Autodesk Inventor part; units mm, degrees
ref_plane "YZ Plane" through (0, 0, 0) normal (1, 0, 0) x (0, 1, 0)
ref_plane "XZ Plane" through (0, 0, 0) normal (0, 1, 0) x (-1, 0, 0)
ref_plane "XY Plane" through (0, 0, 0) normal (0, 0, 1) x (1, 0, 0)
sketch "Sketch1" plane through (0, 0, 0) normal (1, 0, 0) x (0, 1, 0)
  line L0 (-30, 12.5) -> (30, 12.5)
  line L1 (30, 12.5) -> (30, -12.5)
  line L2 (30, -12.5) -> (-30, -12.5)
  line L3 (-30, -12.5) -> (-30, 12.5)
  line L4 (-30, 12.5) -> (30, -12.5) construction
  line L5 (30, 12.5) -> (-30, -12.5) construction
  line L6 (28, -10.5) -> (28, 10.5)
  line L7 (28, 10.5) -> (-28, 10.5)
  line L8 (-28, 10.5) -> (-28, -10.5)
  line L9 (-28, -10.5) -> (28, -10.5)
  point P0 (0, 0)
  dimension "d0" = 60
  dimension "d1" = 25
  dimension "d2" = 2
extrude "Extrusion1" add sketch "Sketch1" along normal blind 70
sketch "Sketch2" plane through (0, 30, 12.5) normal (0, 1, 0) x (1, 0, 0)
  circle A0 centre (15, 12.5) radius 2.75
  circle A1 centre (35, 12.5) radius 2.75
  circle A2 centre (55, 12.5) radius 2.75
  line L0 (0, 0) -> (0, 25)
  line L1 (15, 12.5) -> (55, 12.5) construction
  point P0 (0, 12.5)
  point P1 (0, 12.5)
  dimension "d5" = 5.5
  dimension "d6" = 5.5
  dimension "d7" = 5.5
  dimension "d8" = 20
  dimension "d9" = 20
  dimension "d10" = 15
  dimension "d11" = 40
extrude "Extrusion2" cut sketch "Sketch2" against normal through all
sketch "Sketch3" plane through (0, -30, 12.5) normal (0, 0, 1) x (1, 0, 0)
  circle A0 centre (35, 30) radius 20
  line L0 (70, 60) -> (70, 0)
  line L1 (0, 0) -> (70, 0)
  point P0 (0, 30)
  dimension "d14" = 40
  dimension "d15" = 35
  dimension "d16" = 30
extrude "Extrusion3" cut sketch "Sketch3" against normal blind 30
properties part number "Bumper Support" material "Aluminum 6061"
Input: part model. Units: mm. Frame: model coordinates. A direction names the side the tool comes from. Coordinates: 2 decimals unless noted, no trailing zeros. Order: outer loops, then holes, each group sorted by start corner. A loop starts at its lowest first (then second) coordinate and runs counter-clockwise, first axis right, second up. Notation, with made-up numbers: (34.5, -17.75) - (74.5, -17.75) arc R23 ccw to (74.5, 2.25) - close; hole circle Ø9 at (22.5, 10). An arc over 180 degrees is marked (long way). Put each result on its own line as item: value.
1. Draft query along Z for faces 1 (the face through (34.5, -20.4, 12.5)), 2 (the face through (54.076, 6.007, 11.514)), 3 (the face through (52.253, -28.986, -0.121)). Return one class per face: pulls with the +Z half, pulls with the -Z half, needs draft (parallel to the pull), parting line crosses it, or undercut.
Report:
face 1: pulls with the +Z half
face 2: needs draft
face 3: undercut
2. Contact query for flat-ended pins moving along their axis: pin 1 Ø9 at (x, z) = (35, 0) entering from +Y; pin 2 Ø5 at (x, z) = (15, 0) entering from -Y. Output: stop coordinate, or through.
Report:
pin 1: stops at y = 30
pin 2: passes through
3. Cut plane A-A on y = -23.5. Return the cut outline in (x, z).
Report:
outline: (0, -12.5) - (70, -12.5) - (70, -10.5) - (0, -10.5) - close; (0, 10.5) - (70, 10.5) - (70, 12.5) - (0, 12.5) - close
4. Cut plane D-D on x = 10. Return the cut outline in (y, z).
Report:
outline: (-30, -12.5) - (30, -12.5) - (30, 12.5) - (-30, 12.5) - close; hole (-28, -10.5) - (28, -10.5) - (28, 10.5) - (-28, 10.5) - close
5. Cut plane B-B on x = 35. Return the cut outline in (y, z).
Report:
outline: (-30, -12.5) - (-20, -12.5) - (-20, -10.5) - (-28, -10.5) - (-28, -2.75) - (-30, -2.75) - close; (-30, 2.75) - (-28, 2.75) - (-28, 10.5) - (-20, 10.5) - (-20, 12.5) - (-30, 12.5) - close; (20, -12.5) - (30, -12.5) - (30, -2.75) - (28, -2.75) - (28, -10.5) - (20, -10.5) - close; (20, 10.5) - (28, 10.5) - (28, 2.75) - (30, 2.75) - (30, 12.5) - (20, 12.5) - close
6. Cut plane C-C on z = 4.25. Return the cut outline in (x, y), then the cut area to 3 significant figures.
Report:
outline: (0, -30) - (70, -30) - (70, -28) - (0, -28) - close; (0, 28) - (70, 28) - (70, 30) - (0, 30) - close
area: 280 mm2
7. Line query: line 1 along X through (y, z) = (-29.25, 0); line 2 along Y through (x, z) = (61, 4.5); line 3 along Z through (x, y) = (54.5, -14). Output: solid intervals per line, ascending.
Report:
line 1: x = 0 to 12.25, 17.75 to 32.25, 37.75 to 52.25, 57.75 to 70
line 2: y = -30 to -28, 28 to 30
line 3: z = -12.5 to -10.5, 10.5 to 12.5
8. Reachability of faces 4 (the face through (35, 28, -5)), 5 (the face through (12.253, -28.986, -0.121)) from +Z, -Z, +X, -X, +Y, -Y: full face, straight path, thin tool, end or side. Return the list, or none.
Report:
face 4: +X, -X
face 5: +Y, -Y
